```python
from build123d import *
from OCP.BRepFilletAPI import BRepFilletAPI_MakeChamfer

# Parameters (mm, degrees)
EXTRUDE_1_DEPTH     = 12
SKETCH_2_R          = 3
SKETCH_2_R_2        = 0.81
CUT_EXTRUDE_1_DEPTH = 12
CUT_EXTRUDE_2_DEPTH = 8
FILLET_1_R          = 3
SKETCH_4_R          = 2.25
CUT_EXTRUDE_3_DEPTH = 10
SKETCH_5_W          = 20
SKETCH_5_H          = 63
CUT_EXTRUDE_4_DEPTH = 8
CHAMFER_4_SIZE      = 3.356398525
CHAMFER_4_SIZE_2    = 4
CHAMFER_5_SIZE      = 2


# Some blends are built 0.0001 mm under size
with BuildPart() as part:
    # 草图1 → 凸台-拉伸1 (new body)
    with BuildSketch(Plane(origin=(0, 0, 0), x_dir=(1, 0, 0), z_dir=(0, 1, 0))):
        with BuildLine():
            Line((0, 0), (28, 0))
            ThreePointArc((28, 0), (30.121320344, 0.878679656), (31, 3))
            Line((31, 3), (31, 77))
            Line((31, 77), (-3, 77))
            Line((-3, 77), (-3, 3))
            ThreePointArc((-3, 3), (-2.121320344, 0.878679656), (0, 0))
        make_face()
    extrude(amount=EXTRUDE_1_DEPTH)

    # 草图2 → 切除-拉伸1 (cut)
    with BuildSketch(Plane(origin=(14.000000253, 12, -382.2), x_dir=(1, 0, 0), z_dir=(0, 1, 0))):
        with Locations(Location((13, -352.069110398, 0), (0, 0, 270))):
            Circle(SKETCH_2_R)
        with Locations(Location((-13, -352.069110398, 0), (0, 0, 270))):
            Circle(SKETCH_2_R)
        with Locations(Location((13, -378.069110398, 0), (0, 0, 270))):
            Circle(SKETCH_2_R)
        with Locations(Location((-13, -378.069110398, 0), (0, 0, 270))):
            Circle(SKETCH_2_R)
        with Locations(Location((-15.000000143, -309.999984702, 0), (0, 0, 270))):
            Circle(SKETCH_2_R_2)
        with Locations(Location((15.000000143, -309.999984702, 0), (0, 0, 270))):
            Circle(SKETCH_2_R_2)
        with Locations(Location((14.500000253, -365.000006616, 0), (0, 0, 270))):
            Circle(SKETCH_2_R_2)
        with Locations(Location((-14.500000253, -365.000006616, 0), (0, 0, 270))):
            Circle(SKETCH_2_R_2)
    extrude(amount=-CUT_EXTRUDE_1_DEPTH, mode=Mode.SUBTRACT)

    # 草图3 → 切除-拉伸2 (cut)
    with BuildSketch(Plane(origin=(14.000000253, 12, -382.2), x_dir=(1, 0, 0), z_dir=(0, 1, 0))):
        with BuildLine():
            Line((-7.000000134, -341.834781862), (-7.000000134, -355.639881164))
            ThreePointArc((-7.000000134, -355.639881164), (-7.313370109, -357.994123887), (-8.231657645, -360.184422392))
            ThreePointArc((-8.231657645, -360.184422392), (0, -374.536779603), (8.231657645, -360.184422392))
            ThreePointArc((8.231657645, -360.184422392), (7.313370109, -357.994123887), (7.000000134, -355.639881164))
            Line((7.000000134, -355.639881164), (7.000000134, -341.834782031))
            ThreePointArc((7.000000134, -341.834782031), (3.09e-07, -316.249981647), (-7.000000134, -341.834781862))
        make_face()
    extrude(amount=-CUT_EXTRUDE_2_DEPTH, mode=Mode.SUBTRACT)

    # 圆角1
    fillet_1_edges = [part.edges().sort_by_distance(p)[0] for p in [
        (-3, 6, -77),
        (31, 6, -77),
    ]]
    fillet(fillet_1_edges, radius=FILLET_1_R)

    # 草图4 → 切除-拉伸3 (cut)
    with BuildSketch(Plane.XZ):
        with Locations(Location((-0.5, -17.199993384, 0), (0, 0, 270))):
            Circle(SKETCH_4_R)
        with Locations(Location((28.500000507, -17.199993384, 0), (0, 0, 270))):
            Circle(SKETCH_4_R)
        with Locations((-0.99999989, -72.200015298)):
            Circle(SKETCH_4_R)
        with Locations((29.000000396, -72.200015298)):
            Circle(SKETCH_4_R)
    extrude(amount=-CUT_EXTRUDE_3_DEPTH, mode=Mode.SUBTRACT)

    # 草图5 → 切除-拉伸4 (cut)
    with BuildSketch(Plane.XZ):
        Polygon((28, -77), (0, -77), (-3, -77), (-3, -71.169239105), (-3, -3), (-3, 0), (0, 0), (28, 0), (31, 0), (31, -3), (31, -71.169238122), (31, -77), align=None)
        with Locations((14, -38.5)):
            Rectangle(SKETCH_5_W, SKETCH_5_H, mode=Mode.SUBTRACT)
    extrude(amount=-CUT_EXTRUDE_4_DEPTH, mode=Mode.SUBTRACT)

    # 倒角4
    chamfer_4_edges_1 = [part.edges().sort_by_distance(p)[0] for p in [
        (24, 0, -38.5),
    ]]
    chamfer_4_side_1 = [part.faces().sort_by_distance(p)[0] for p in [
        (23.93287203, 0, -38.5),
    ]]
    chamfer_4_edges_2 = [part.edges().sort_by_distance(p)[0] for p in [
        (4, 0, -38.5),
    ]]
    chamfer_4_side_2 = [part.faces().sort_by_distance(p)[0] for p in [
        (4.06712797, 0, -38.5),
    ]]
    chamfer_4_edges_3 = [part.edges().sort_by_distance(p)[0] for p in [
        (14, 0, -7),
    ]]
    chamfer_4_side_3 = [part.faces().sort_by_distance(p)[0] for p in [
        (14, 0, -7.06712797),
    ]]
    chamfer_4_edges_4 = [part.edges().sort_by_distance(p)[0] for p in [
        (14, 0, -70),
    ]]
    chamfer_4_side_4 = [part.faces().sort_by_distance(p)[0] for p in [
        (14, 0, -69.93287203),
    ]]
    chamfer_4 = BRepFilletAPI_MakeChamfer(part.part.solid().wrapped)
    for e in chamfer_4_edges_1:
        chamfer_4.Add(CHAMFER_4_SIZE - 0.0001, CHAMFER_4_SIZE_2 - 0.0001, e.wrapped, chamfer_4_side_1[0].wrapped)
    for e in chamfer_4_edges_2:
        chamfer_4.Add(CHAMFER_4_SIZE - 0.0001, CHAMFER_4_SIZE_2 - 0.0001, e.wrapped, chamfer_4_side_2[0].wrapped)
    for e in chamfer_4_edges_3:
        chamfer_4.Add(CHAMFER_4_SIZE - 0.0001, CHAMFER_4_SIZE_2 - 0.0001, e.wrapped, chamfer_4_side_3[0].wrapped)
    for e in chamfer_4_edges_4:
        chamfer_4.Add(CHAMFER_4_SIZE - 0.0001, CHAMFER_4_SIZE_2 - 0.0001, e.wrapped, chamfer_4_side_4[0].wrapped)
    add(Compound.cast(chamfer_4.Shape()), mode=Mode.REPLACE)  # a hair under: the kernel refuses the full size

    # 倒角5
    # the kernel refuses this chamfer: 2 mm, written as the material it takes off along each edge
    with BuildSketch(Plane(origin=(28, 8, 0), x_dir=(0, -0.027495876610586494, -0.9996219169112968), z_dir=(-1, 0, 0)), Plane(origin=(0, 8, -77), x_dir=(0, -0.027495876610586414, 0.9996219169112968), z_dir=(1, 0, 0))) as chamfer_5_piece_1:
        Polygon((CHAMFER_5_SIZE * 0.999621916911, -CHAMFER_5_SIZE * 0.0274958766106), (-CHAMFER_5_SIZE * 0.0274958766106, -CHAMFER_5_SIZE * 0.999621916911), (0, 0), align=None)
    extrude(amount=28, mode=Mode.SUBTRACT)
    with BuildSketch(Plane(origin=(31, 8, -76.312604098), x_dir=(-0.9996219169112968, -0.02749587661058651, 0), z_dir=(0, 0, 1))) as chamfer_5_piece_2:
        Polygon((CHAMFER_5_SIZE * 0.999621916911, -CHAMFER_5_SIZE * 0.0274958766106), (-CHAMFER_5_SIZE * 0.0274958766106, -CHAMFER_5_SIZE * 0.999621916911), (0, 0), align=None)
    extrude(amount=73.312604098, mode=Mode.SUBTRACT)
    with BuildSketch(Plane(origin=(-3, 8, -68.087425514), x_dir=(0.9996219169112968, -0.027495876610586487, 0), z_dir=(0, 0, -1))) as chamfer_5_piece_3:
        Polygon((CHAMFER_5_SIZE * 0.999621916911, -CHAMFER_5_SIZE * 0.0274958766106), (-CHAMFER_5_SIZE * 0.0274958766106, -CHAMFER_5_SIZE * 0.999621916911), (0, 0), align=None)
    extrude(amount=5.912574486, mode=Mode.SUBTRACT)
    with BuildSketch(Plane(origin=(31, 8, -74), x_dir=(-0.9996219169112968, -0.02749587661058651, 0), z_dir=(0, 0, 1))) as chamfer_5_piece_4:
        Polygon((CHAMFER_5_SIZE * 0.999621916911, -CHAMFER_5_SIZE * 0.0274958766106), (-CHAMFER_5_SIZE * 0.0274958766106, -CHAMFER_5_SIZE * 0.999621916911), (0, 0), align=None)
    extrude(amount=5.912573503, mode=Mode.SUBTRACT)
    with BuildSketch(Plane(origin=(0, 8, -74), x_dir=(0, 0, -1), z_dir=(1, 0, 0))) as chamfer_5_piece_5:
        Polygon((3 - CHAMFER_5_SIZE, 0), (3, CHAMFER_5_SIZE), (3, 0), align=None)
    revolve(axis=Axis((0, 8, -74), (0, 1, 0)), revolution_arc=90, mode=Mode.SUBTRACT)
    with BuildSketch(Plane(origin=(28, 8, -74), x_dir=(1, 0, 0), z_dir=(0, 0, 1))) as chamfer_5_piece_6:
        Polygon((3 - CHAMFER_5_SIZE, 0), (3, CHAMFER_5_SIZE), (3, 0), align=None)
    revolve(axis=Axis((28, 8, -74), (0, 1, 0)), revolution_arc=90, mode=Mode.SUBTRACT)
    with BuildSketch(Plane(origin=(28, 8, -3), x_dir=(1, 0, 0), z_dir=(0, 0, -1))) as chamfer_5_piece_7:
        Polygon((3 - CHAMFER_5_SIZE, 0), (3, -CHAMFER_5_SIZE), (3, 0), align=None)
    revolve(axis=Axis((28, 8, -3), (0, -1, 0)), revolution_arc=90, mode=Mode.SUBTRACT)
    with BuildSketch(Plane(origin=(0, 8, -3), x_dir=(0, 0, 1), z_dir=(1, 0, 0))) as chamfer_5_piece_8:
        Polygon((3 - CHAMFER_5_SIZE, 0), (3, -CHAMFER_5_SIZE), (3, 0), align=None)
    revolve(axis=Axis((0, 8, -3), (0, -1, 0)), revolution_arc=90, mode=Mode.SUBTRACT)
    with BuildSketch(Plane(origin=(-3, 8, -3), x_dir=(0.9996219169112968, -0.027495876610586497, 0), z_dir=(0, 0, -1))) as chamfer_5_piece_9:
        Polygon((CHAMFER_5_SIZE * 0.999621916911, -CHAMFER_5_SIZE * 0.0274958766106), (-CHAMFER_5_SIZE * 0.0274958766106, -CHAMFER_5_SIZE * 0.999621916911), (0, 0), align=None)
    extrude(amount=73.312605081, mode=Mode.SUBTRACT)


solid = part.part
```
For this review, take the finished solid that the model builds, in its own axes (mm). A direction names the side the tool comes from. Coordinates: 2 decimals unless noted, no trailing zeros. Loops run counter-clockwise (first coordinate to the right, second up) from the corner with the lowest first, then second, coordinate; pieces in that order, holes last. Notation, with made-up numbers: (-30, 20.5) - (25, 20.5) arc R8 cw to (25, 35.5) - close; hole circle Ø11 at (87.25, -21.75). An arc over 180 degrees is marked (long way). Use one line per item in the form item = value. Start each with the question number.
1) To check wall thickness, follow probe 1 along X at (y, z) = (7.5, -27.5); probe 2 along Z at (x, y) = (14, 7); probe 3 along Y at (x, z) = (26, -63). State the ranges of each line that lie inside material, in increasing order. Write a range as from..to.
2) Take a section at D-D (z = -5). State the section outline as (x, y) points, plus the area to 3 significant figures.
3) Draft analysis for pull direction X (two halves, no side actions). For faces 4 (the face through (-2, 10, -72)), 5 (the face through (29.44, 9.014, -75.408)), 6 (the face through (14, 9, -1)), state which applies: released by +X, released by -X, zero draft, split by the parting line, or undercut.
4) Take a section at B-B (z = -34). State the section outline as (x, y) points.
5) Take a section at A-A (y = 7). State the section outline as (x, z) points, plus the area to 3 significant figures.
6) For faces 1 (the face through (7, 8, -34)), 2 (the face through (14, 6, -70)), 3 (the face through (1.73, 9.25, -16.91)), list the 3-axis set-ups (+Z, -Z, +X, -X, +Y, -Y) from which the entire face can be reached by the end or side of a thin tool; tool diameter is ignored.
7) For pin 1 (3 mm diameter, centred on y = 5, z = -37, fed in from +X); pin 2 (1.5 mm diameter, centred on y = 8, z = -41.5, fed in from +X); pin 3 (4 mm diameter, centred on x = 5, y = 1.5, fed in from +Z); pin 4 (1.3 mm diameter, centred on x = -0.5, z = -17.2, fed in from -Y), all flat-tipped, find the tip position at first contact; note any pin that passes through.
8) Take a section at C-C (x = 14). State the section outline as (y, z) points, plus the area to 3 significant figures.
From the geometry:
q1.probe_1 = 4..7, 21..24
q1.probe_2 = -70..-65.95, -7.66..-7
q1.probe_3 = 8..12
q2.outline = (-3, 10) - (-1.87, 8.87) - (-1.87, 12) - (-3, 12) - close; (3.87, 8) - (24.13, 8) - (24.13, 12) - (3.87, 12) - close; (29.87, 8.87) - (31, 10) - (31, 12) - (29.87, 12) - close
q2.area = 86.8 mm2
q3.face_4 = undercut
q3.face_5 = released by +X
q3.face_6 = zero draft
q4.outline = (-3, 10) - (-1, 8) - (4, 8) - (4, 4) - (7.36, 0) - (20.64, 0) - (24, 4) - (24, 8) - (29, 8) - (31, 10) - (31, 12) - (21, 12) - (21, 4) - (7, 4) - (7, 12) - (-3, 12) - close
q5.outline = (4, -70) - (24, -70) - (24, -61.64) arc R13.75 cw to (4, -61.64) - close; (4, -42.76) arc R13.75 cw to (7, -40.37) - (7, -26.56) arc R9 ccw to (5.77, -22.02) arc R9.54 cw (long way) to (22.23, -22.02) arc R9 ccw to (21, -26.56) - (21, -40.37) arc R13.75 cw to (24, -42.76) - (24, -7) - (4, -7) - close
q5.area = 290 mm2
q6.face_1 = +Y
q6.face_2 = -Z, +X, -X, -Y
q6.face_3 = -Y
q7.pin_1 = 24
q7.pin_2 = 29.75
q7.pin_3 = -7.42
q7.pin_4 = through
q8.outline = (0, -66.64) - (4, -70) - (8, -70) - (8, -75) - (10, -77) - (12, -77) - (12, -65.95) - (4, -65.95) - (4, -7.66) - (12, -7.66) - (12, 0) - (10, 0) - (8, -2) - (8, -7) - (4, -7) - (0, -10.36) - close
q8.area = 328 mm2
